Geometry: final body of the model. Coordinates: model frame, mm. Coordinates: 2 decimals unless noted, no trailing zeros. Order: outer loops, then holes, each group sorted by start corner. A loop starts at its lowest first (then second) coordinate and runs counter-clockwise, first axis right, second up. Notation, with made-up numbers: (13.25, 66) - (64.25, 66) arc R13 ccw to (64.25, 76) - close; hole circle Ø8 at (77.25, -35.5). An arc over 180 degrees is marked (long way). Use a Markdown table: item, result. Add a question column.
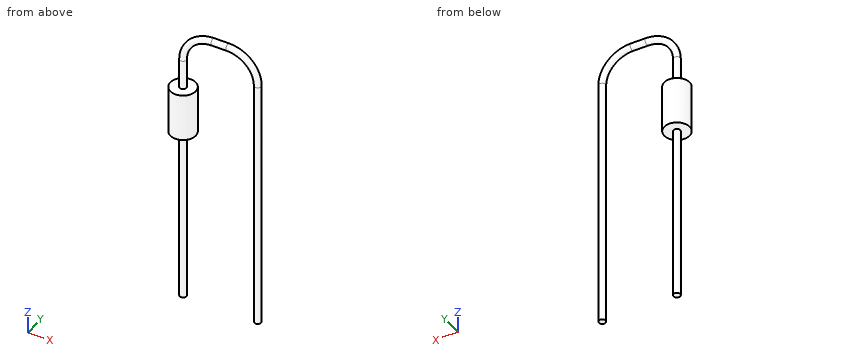
```python
from build123d import *

# Parameters (mm, degrees)
SKETCH2_R           = 0.85
RESISTOR_BODY_DEPTH = 3.2
LEAD1_PROFILE_R     = 0.225
SKETCH6_R           = 0.225
LEAD2_DEPTH         = 11.8


with BuildPart() as part:
    # Sketch2 → Resistor Body (new body)
    with BuildSketch(Plane.XY):
        Circle(SKETCH2_R)
    extrude(amount=RESISTOR_BODY_DEPTH)

    # Lead1: sweep along a path in Lead1 Path
    with BuildLine(Plane.XZ) as lead1_path:
        Line((0, 3.2), (0, 5.2))
        ThreePointArc((0, 5.2), (0.585786438, 6.614213562), (2, 7.2))
        Line((2, 7.2), (3, 7.2))
        ThreePointArc((3, 7.2), (4.414213562, 6.614213562), (5, 5.2))
        Line((5, 5.2), (5, -11.8))
    # Lead1 Profile → Lead1 (sweep)
    with BuildSketch(Plane(origin=(0, 0, 3.2), x_dir=(-1, 0, 0), z_dir=(0, 0, 1))):
        Circle(LEAD1_PROFILE_R)
    sweep(path=lead1_path.line)

    # Sketch6 → Lead2 (add)
    with BuildSketch(Plane(origin=(0, 0, 0), x_dir=(1, 0, 0), z_dir=(0, 0, -1))):
        Circle(SKETCH6_R)
    extrude(amount=LEAD2_DEPTH)


solid = part.part
```
1) First-contact query: pin 1 (0.5 mm diameter, centred on x = -0.5, y = 0.5, fed in from +Z); pin 2 (1 mm diameter, centred on x = 1, z = 3, fed in from -Y). Flat tips, straight axial feed; report the tip coordinate or a pass-through.
2) Section query B-B (y = 0). Return the cut outline in (x, z) (3 decimals).
3) Line query: line 1 (X direction, y = 0.1, z = -9.5); line 2 (Z direction, x = -0.5, y = -0.55); line 3 (X direction, y = -0.3, z = 2). Output: solid intervals per line, ascending. Write a range as from..to.
4) Section query A-A (z = 1). Return the cut outline in (x, y) (3 decimals).
5) Section query C-C (z = -1.5). Return the cut outline in (x, y) (3 decimals), and give its area (3 significant figures).
6) Section query D-D (x = 2.25). Return the cut outline in (y, z) (3 decimals).
From the geometry:
| question | item | result |
|---|---|---|
| 1 | pin 1 | stops at z = 3.2 |
| 1 | pin 2 | stops at y = -0.69 |
| 2 | outline | (-0.85, 0) - (-0.225, 0) - (-0.225, -11.8) - (0.225, -11.8) - (0.225, 0) - (0.85, 0) - (0.85, 3.2) - (0.225, 3.2) - (0.225, 5.2) arc R1.775 cw to (2, 6.975) - (3, 6.975) arc R1.775 cw to (4.775, 5.2) - (4.775, -11.8) - (5.225, -11.8) - (5.225, 5.2) arc R2.225 ccw to (3, 7.425) - (2, 7.425) arc R2.225 ccw to (-0.225, 5.2) - (-0.225, 3.2) - (-0.85, 3.2) - close |
| 3 | line 1 | x = -0.2..0.2, 4.8..5.2 |
| 3 | line 2 | z = 0..3.2 |
| 3 | line 3 | x = -0.8..0.8 |
| 4 | outline | circle Ø1.7 at (0, 0); circle Ø0.45 at (5, 0) |
| 5 | outline | circle Ø0.45 at (0, 0); circle Ø0.45 at (5, 0) |
| 5 | area | 0.318 mm^2 |
| 6 | outline | circle Ø0.45 at (0, 7.2) |
